The listing builds one solid part. Answer for the finished solid, in the listing's coordinates (mm). A direction names the side the tool comes from. Coordinates: 2 decimals unless noted, no trailing zeros. Loops run counter-clockwise (first coordinate to the right, second up) from the corner with the lowest first, then second, coordinate; pieces in that order, holes last. Notation, with made-up numbers: (-24.5, -8) - (20.5, -8) arc R21 cw to (20.5, -2) - close; hole circle Ø8 at (3.5, 63). An arc over 180 degrees is marked (long way). One line per question, with ' | ' between items.
from build123d import *
from build123d import SkipClean  # not in build123d's __all__

# Parameters (mm, degrees)
F1_DEPTH = 5
F2_R     = 0.7


with BuildPart() as f1:
    # F0 (on Front) → F1 (new body)
    with BuildSketch(Plane.XZ):
        with BuildLine():
            Line((0, -1), (0, 0))
            Line((0, 0), (-28.0174232112, 0))
            Line((-28.0174232112, 0), (-28.4, 7.3))
            ThreePointArc((-28.4, 7.3), (-34.4838071024, 11.365069943), (-35.9112698372, 4.1887301628))
            Line((-35.9112698372, 4.1887301628), (-34.4970562748, 5.6029437252))
            ThreePointArc((-34.4970562748, 5.6029437252), (-33.7184402377, 9.517310878), (-30.4, 7.3))
            Line((-30.4, 7.3), (-29.7920697603, -4.3))
            Line((-29.7920697603, -4.3), (0, -4.3))
            Line((0, -4.3), (0, -3.3))
            ThreePointArc((0, -3.3), (-1.15, -2.15), (0, -1))
        make_face()
    extrude(amount=F1_DEPTH)

    # F2
    f2_edges = [f1.edges().sort_by_distance(p)[0] for p in [
        (-28.017423, -2.5, 0),
        (-29.79207, -2.5, -4.3),
        (-34.497056, -2.5, 5.602944),
        (-35.91127, -2.5, 4.18873),
    ]]
    fillet(f2_edges, radius=F2_R)

    # F3: F1 across plane


with BuildPart() as f1_1:
    add(f1.part, clean=False)
    with SkipClean():  # cleaning this boolean's faces spoils the solid; the shape is the same uncleaned
        add(f1.part.mirror(Plane.YZ), clean=False)


solid = f1_1.part
Item 1: Find section B-B, the plane z = -2.15. Write down the section's boundary in (x, y), plus the area to 3 significant figures.
Taken from the geometry:
outline: (-29.9, -5) - (-1.15, -5) - (-1.15, 0) - (-29.9, 0) - close; (1.15, -5) - (29.9, -5) - (29.9, 0) - (1.15, 0) - close | area: 288 mm2
Item 2: Find section C-C, the plane z = 9. Write down the section's boundary in (x, y).
Taken from the geometry:
outline: (-36.86, -5) - (-34.49, -5) - (-34.49, 0) - (-36.86, 0) - close; (-31.11, -5) - (-28.74, -5) - (-28.74, 0) - (-31.11, 0) - close; (28.74, -5) - (31.11, -5) - (31.11, 0) - (28.74, 0) - close; (34.49, -5) - (36.86, -5) - (36.86, 0) - (34.49, 0) - close
Item 3: Find section D-D, the plane y = -0.7. Write down the section's boundary in (x, z), plus the area to 3 significant figures.
Taken from the geometry:
outline: (-36.44, 4.83) arc R0.7 ccw to (-35.37, 4.73) - (-34.94, 5.16) arc R0.7 ccw to (-34.84, 6.03) arc R2.4 cw (long way) to (-30.4, 7.3) - (-29.83, -3.64) arc R0.7 ccw to (-29.13, -4.3) - (29.13, -4.3) arc R0.7 ccw to (29.83, -3.64) - (30.4, 7.3) arc R2.4 cw (long way) to (34.84, 6.03) arc R0.7 ccw to (34.94, 5.16) - (35.37, 4.73) arc R0.7 ccw to (36.44, 4.83) arc R4.4 ccw (long way) to (28.4, 7.3) - (28.05, 0.66) arc R0.7 cw to (27.35, 0) - (-27.35, 0) arc R0.7 cw to (-28.05, 0.66) - (-28.4, 7.3) arc R4.4 ccw (long way) to start; hole circle Ø2.3 at (0, -2.15) | area: 335 mm2
Item 4: This flat-tipped pin is pushed along its axis until it touches: pin 1 Ø2 at (y, z) = (-2, 3) entering from +X. Where does it stop, or does it pass through?
Taken from the geometry:
pin 1: stops at x = 30.23
Item 5: The mould has two halves that part along X. Classify faces 4 (the face through (33.52, -2.46, 9.59)), 5 (the face through (0, -2, -4.3)): pulls with the +X half, pulls with the -X half, needs draft (parallel to the pull), parting line crosses it, or undercut.
Taken from the geometry:
face 4: undercut | face 5: needs draft
Item 6: Which of the six approach directions +Z, -Z, +X, -X, +Y, -Y give full straight-line access (tool end or side, diameter ignored) to faces 1 (the face through (-30.117, -2.465, 1.908)), 2 (the face through (-2.6, -5, -0.4)), 3 (the face through (0, -2, 0))?
Taken from the geometry:
face 1: -Z, +Y, -Y | face 2: +Z, -Z, +X, -X, -Y | face 3: +Z, +Y, -Y
Item 7: Find the intervals of material crossed by line 1 (X direction, y = -1.6, z = 7.3); line 2 (X direction, y = -4.05, z = 6); line 3 (Z direction, x = 32.8, y = -2.3), in increasing order. Write a range as [from, to].
Taken from the geometry:
line 1: x = [-37.2, -35.2], [-30.4, -28.4], [28.4, 30.4], [35.2, 37.2] | line 2: x = [-37, -34.82], [-30.33, -28.33], [28.33, 30.33], [34.82, 37] | line 3: z = [9.7, 11.7]
Item 8: Find section A-A, the plane x = 0. Write down the section's boundary in (y, z), plus the area to 4 significant figures.
Taken from the geometry:
outline: (-5, -4.3) - (0, -4.3) - (0, -3.3) - (-5, -3.3) - close; (-5, -1) - (0, -1) - (0, 0) - (-5, 0) - close | area: 10.00 mm2
